```python
from build123d import *

# Parameters (mm, degrees)
F0_W      = 42
F0_H      = 42
F1_DEPTH  = 10
F2_SIZE   = 4
F3_R      = 16.5
F4_DEPTH  = 0.5
F5_R      = 11
F6_DEPTH  = 2.5
F7_R      = 3.5
F8_DEPTH  = 12.001
F9_R      = 2
F10_SIZE  = 0.5
F12_DEPTH = 3
F13_R     = 1.5
F14_DEPTH = 10.001


with BuildPart() as f1:
    # F0 (on Front) → F1 (new body)
    with BuildSketch(Plane.XZ):
        Rectangle(F0_W, F0_H)
    extrude(amount=F1_DEPTH)

    # F2
    f2_edges = [f1.edges().sort_by_distance(p)[0] for p in [
        (-21, -5, 21),
        (21, -5, 21),
        (21, -5, -21),
        (-21, -5, -21),
    ]]
    chamfer(f2_edges, length=F2_SIZE)

    # F3 (on face) → F4 (cut)
    with BuildSketch(Plane.XZ.offset(10)):
        Circle(F3_R)
    extrude(amount=-F4_DEPTH, mode=Mode.SUBTRACT)

    # F5 (on face) → F6 (join)
    with BuildSketch(Plane.XZ.offset(9.5)):
        Circle(F5_R)
    extrude(amount=F6_DEPTH)

    # F7 (on face) → F8 (cut, through all)
    with BuildSketch(Plane.XZ.offset(12)):
        Circle(F7_R)
    extrude(amount=-F8_DEPTH, mode=Mode.SUBTRACT)

    # F9
    f9_edges = [f1.edges().sort_by_distance(p)[0] for p in [
        (-17, -5, 21),
        (17, -5, 21),
        (21, -5, 17),
        (21, -5, -17),
        (17, -5, -21),
        (-17, -5, -21),
        (-21, -5, -17),
        (-21, -5, 17),
    ]]
    fillet(f9_edges, radius=F9_R)

    # F10
    f10_edges = [f1.edges().sort_by_distance(p)[0] for p in [
        (-11, -12, 0),
        (-3.5, -12, 0),
        (-11, -9.5, 0),
    ]]
    chamfer(f10_edges, length=F10_SIZE)

    # F11 (on face) → F12 (cut)
    with BuildSketch(Plane(origin=(0, 0, 0), x_dir=(-1, 0, 0), z_dir=(0, 1, 0))):
        with BuildLine():
            ThreePointArc((-14.5105618091, 21), (-17.8908729653, 17.8908729653), (-21, 14.5105618091))
            Line((-21, 14.5105618091), (-21, -14.5105618091))
            ThreePointArc((-21, -14.5105618091), (-17.8908729653, -17.8908729653), (-14.5105618091, -21))
            Line((-14.5105618091, -21), (14.5105618091, -21))
            ThreePointArc((14.5105618091, -21), (17.8908729653, -17.8908729653), (21, -14.5105618091))
            Line((21, -14.5105618091), (21, 14.5105618091))
            ThreePointArc((21, 14.5105618091), (17.8908729653, 17.8908729653), (14.5105618091, 21))
            Line((14.5105618091, 21), (-14.5105618091, 21))
        make_face()
    extrude(amount=-F12_DEPTH, mode=Mode.SUBTRACT)

    # F13 (on face) → F14 (cut, through all)
    with BuildSketch(Plane.XZ.offset(10)):
        with Locations((-15.5, 15.5)):
            Circle(F13_R)
        with Locations((-15.5, -15.5)):
            Circle(F13_R)
        with Locations((15.5, -15.5)):
            Circle(F13_R)
        with Locations((15.5, 15.5)):
            Circle(F13_R)
    extrude(amount=-F14_DEPTH, mode=Mode.SUBTRACT)


solid = f1.part
```
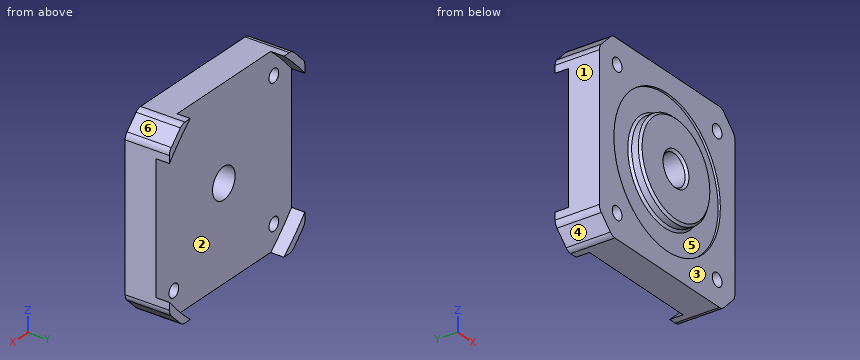
Verification items for the finished model (mm, model axes). Face numbers are marked on the shaded views. A direction names the side the tool comes from. Give positions to 0.01 mm unless a question says otherwise; leave off trailing zeros. Order: outer loops, then holes, each group sorted by start corner. A loop starts at its lowest first (then second) coordinate and runs counter-clockwise, first axis right, second up. Notation, with made-up numbers: M 2.25,29 L 54.25,29 A17 cw 54.25,54 Z; hole C 80,-7.75 d10. An arc over 180 degrees is marked long. Answer in a Markdown table with one row per item. Add a question column.
Item 1: Section check D-D, the plane x = -15.5. Enter the section's corners in (y, z), and give its area (3 significant figures).
Item 2: Section check A-A, the plane x = 0. Enter the section's corners in (y, z), and give its area (3 significant figures).
Item 3: Section check B-B, the plane z = 0. Enter the section's corners in (x, y), and give its area (3 significant figures).
Item 4: Gauge pin test, flat ends, axial feed: pin 1 (8 mm diameter, centred on x = -11, z = 7, fed in from +Y); pin 2 (4 mm diameter, centred on y = -2, z = -7, fed in from -X); pin 3 (5 mm diameter, centred on x = -15.5, z = 15.5, fed in from -Y). Record the tip position at first contact, or that the pin passes through.
Item 5: Mould release check, pull along X, two halves, no side actions. Record for the marked faces 4, 5 and 6: released by +X, released by -X, zero draft, split by the parting line, or undercut.
Item 6: Tool access check on the marked faces 1, 2 and 3. Record the directions out of +Z, -Z, +X, -X, +Y, -Y that give a thin tool (end or side, any length) a straight path to the whole face; none if there is none.
Item 7: Scan lines: probe 1 along Z at (x, y) = (15.5, -8.25); probe 2 along Z at (x, y) = (0, -6.5); probe 3 along Z at (x, y) = (-2.5, -6.25). Record each from-to range of solid material in increasing order. Write a range as from..to.
Item 8: Section check C-C, the plane y = -1. Enter the section's corners in (x, z), and give its area (3 significant figures).
Filled sheet:
| question | item | result |
|---|---|---|
| 1 | outline | M -10,-21 L 0,-21 L 0,-20.14 L -3,-20.14 L -3,-17 L -10,-17 Z; M -10,-14 L -3,-14 L -3,14 L -10,14 L -10,5.66 L -9.5,5.66 L -9.5,-5.66 L -10,-5.66 Z; M -10,17 L -3,17 L -3,20.14 L 0,20.14 L 0,21 L -10,21 Z |
| 1 | area | 251 mm^2 |
| 2 | outline | M -12,-10.5 L -11.5,-11 L -10,-11 L -9.5,-11.5 L -9.5,-16.5 L -10,-16.5 L -10,-21 L -3,-21 L -3,-3.5 L -11.5,-3.5 L -12,-4 Z; M -12,4 L -11.5,3.5 L -3,3.5 L -3,21 L -10,21 L -10,16.5 L -9.5,16.5 L -9.5,11.5 L -10,11 L -11.5,11 L -12,10.5 Z |
| 2 | area | 269 mm^2 |
| 3 | outline | M -21,-10 L -16.5,-10 L -16.5,-9.5 L -11.5,-9.5 L -11,-10 L -11,-11.5 L -10.5,-12 L -4,-12 L -3.5,-11.5 L -3.5,-3 L -21,-3 Z; M 3.5,-11.5 L 4,-12 L 10.5,-12 L 11,-11.5 L 11,-10 L 11.5,-9.5 L 16.5,-9.5 L 16.5,-10 L 21,-10 L 21,-3 L 3.5,-3 Z |
| 3 | area | 269 mm^2 |
| 4 | pin 1 | stops at y = -3 |
| 4 | pin 2 | stops at x = -21 |
| 4 | pin 3 | stops at y = -10 |
| 5 | face 4 | released by -X |
| 5 | face 5 | undercut |
| 5 | face 6 | released by +X |
| 6 | face 1 | +Z, -Z, -X, +Y, -Y |
| 6 | face 2 | +Y |
| 6 | face 3 | -Y |
| 7 | probe 1 | z = -21..-17, -14..14, 17..21 |
| 7 | probe 2 | z = -21..-3.5, 3.5..21 |
| 7 | probe 3 | z = -21..-2.45, 2.45..21 |
| 8 | outline | M -21,-16.17 A2 ccw -20.41,-17.59 L -17.59,-20.41 A2 ccw -16.17,-21 L -14.51,-21 A55 cw -21,-14.51 Z; M -21,14.51 A55 cw -14.51,21 L -16.17,21 A2 ccw -17.59,20.41 L -20.41,17.59 A2 ccw -21,16.17 Z; M 14.51,-21 L 16.17,-21 A2 ccw 17.59,-20.41 L 20.41,-17.59 A2 ccw 21,-16.17 L 21,-14.51 A55 cw Z; M 14.51,21 A55 cw 21,14.51 L 21,16.17 A2 ccw 20.41,17.59 L 17.59,20.41 A2 ccw 16.17,21 Z |
| 8 | area | 46.8 mm^2 |
